Verification items for the finished model (mm, model axes). Face numbers are marked on the shaded views. A direction names the side the tool comes from. Round coordinates to 2 decimals unless told otherwise and drop trailing zeros. Write each loop counter-clockwise with the first axis right and the second up, starting at its lowest first coordinate (ties: lowest second). Pieces come first, ordered by that corner, then holes.
from build123d import *

# Parameters (mm, degrees)
F0_W     = 30
F0_H     = 12
F1_DEPTH = 5
F2_W     = 30
F2_H     = 7.47772
F3_DEPTH = 4
F4_W     = 15
F4_H     = 7.47772
F4_W_2   = 7
F5_DEPTH = 1.5
F6_W     = 13
F6_H     = 5.47772
F6_W_2   = 5
F7_DEPTH = 2.5
F8_R     = 1.5
F9_DEPTH = 2.5


with BuildPart() as f1:
    # F0 (on Front) → F1 (new body)
    with BuildSketch(Plane.XZ):
        Rectangle(F0_W, F0_H)
    extrude(amount=F1_DEPTH)

    # F2 (on face) → F3 (join)
    with BuildSketch(Plane.XZ.offset(5)):
        Rectangle(F2_W, F2_H)
    extrude(amount=F3_DEPTH)

    # F4 (on face) → F5 (join)
    with BuildSketch(Plane.XZ.offset(9)):
        with Locations((-7.5, 0)):
            Rectangle(F4_W, F4_H)
        with Locations((10.5, 0)):
            Rectangle(F4_W_2, F4_H)
    extrude(amount=F5_DEPTH)

    # F6 (on face) → F7 (cut)
    with BuildSketch(Plane.XZ.offset(10.5)):
        with Locations((-7.5, 0)):
            Rectangle(F6_W, F6_H)
        with Locations((10.5, 0)):
            Rectangle(F6_W_2, F6_H)
    extrude(amount=-F7_DEPTH, mode=Mode.SUBTRACT)

    # F8 (on face) → F9 (join)
    with BuildSketch(Plane(origin=(0, 0, 0), x_dir=(-1, 0, 0), z_dir=(0, 1, 0))):
        with BuildLine():
            Line((-15, 3.5), (-18.5, 3.5))
            ThreePointArc((-18.5, 3.5), (-22, 0), (-18.5, -3.5))
            Line((-18.5, -3.5), (-15, -3.5))
            Line((-15, -3.5), (-15, 3.5))
        make_face()
        with Locations((-18.5, 0)):
            Circle(F8_R, mode=Mode.SUBTRACT)
        with BuildLine():
            Line((18.5, 3.5), (15, 3.5))
            Line((15, 3.5), (15, -3.5))
            Line((15, -3.5), (18.5, -3.5))
            ThreePointArc((18.5, -3.5), (22, 0), (18.5, 3.5))
        make_face()
        with Locations((18.5, 0)):
            Circle(F8_R, mode=Mode.SUBTRACT)
    extrude(amount=-F9_DEPTH)


solid = f1.part
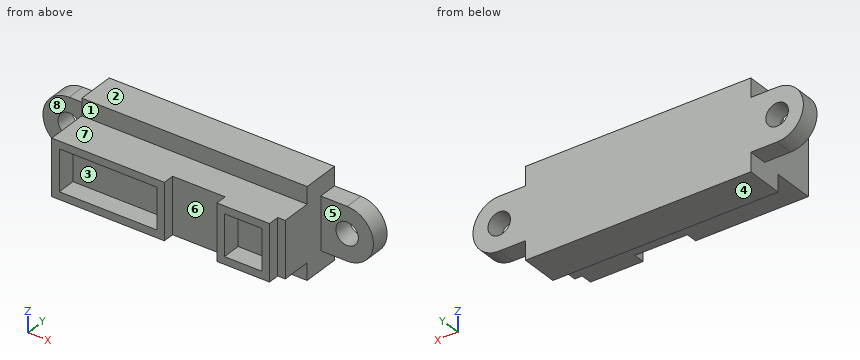
Q1. Material ranges on line 1 along X through (y, z) = (-1.75, -0.5); line 2 along Z through (x, y) = (18.5, -1.9); line 3 along X through (y, z) = (-5, -2), recorded low to high.
Recorded:
line 1: x = -21.96 to -19.91, -17.09 to 17.09, 19.91 to 21.96
line 2: z = -3.5 to -1.5, 1.5 to 3.5
line 3: x = -15 to 15
Q2. Release check for a two-part mould opening along Z. For the marked faces 1, 2, 3 and 4 record: released by +Z, released by -Z, zero draft, split by the parting line, or undercut.
Recorded:
face 1: zero draft
face 2: released by +Z
face 3: undercut
face 4: released by -Z
Q3. Sectioned sample at D-D (x = -6.5). Enter the section's corners in (y, z).
Recorded:
outline: (-10.5, -3.74) - (-5, -3.74) - (-5, -6) - (0, -6) - (0, 6) - (-5, 6) - (-5, 3.74) - (-10.5, 3.74) - (-10.5, 2.74) - (-8, 2.74) - (-8, -2.74) - (-10.5, -2.74) - close
Q4. Sectioned sample at A-A (z = 0). Give the number of separate pieces and of enclosed holes in the cut face, plus the area to 3 significant figures.
Recorded:
separate pieces: 3
enclosed holes: 0
area: 278 mm2
Q5. Depth check by flat-ended pin: P1, Ø3, axis at x = 11, z = 0, coming from the -Y side; P2, Ø1.2, axis at x = -5.5, y = -9.5, coming from the -Z side; P3, Ø1.6, axis at y = -10, z = 0.5, coming from the -X side; P4, Ø2.5, axis at x = 18.5, z = 0, coming from the +Y side. Enter the tip coordinate at first touch or a pass-through.
Recorded:
P1: stops at y = -8
P2: stops at z = -3.74
P3: stops at x = -15
P4: passes through
Q6. Sectioned sample at C-C (x = -19). Enter the section's corners in (y, z), plus the area to 3 significant figures.
Recorded:
outline: (-2.5, -3.46) - (0, -3.46) - (0, -1.41) - (-2.5, -1.41) - close; (-2.5, 1.41) - (0, 1.41) - (0, 3.46) - (-2.5, 3.46) - close
area: 10.2 mm2
Q7. Tool access check on the marked faces 5, 6, 7 and 8. Record the directions out of +Z, -Z, +X, -X, +Y, -Y that give a thin tool (end or side, any length) a straight path to the whole face; none if there is none.
Recorded:
face 5: +Z, -Z, +X, -Y
face 6: +Z, -Z, -Y
face 7: +Z, +X, -X, -Y
face 8: +Z, -Z, -X, -Y
Q8. Sectioned sample at B-B (y = -2). Enter the section's corners in (x, z).
Recorded:
outline: (-18.5, -3.5) - (-15, -3.5) - (-15, -6) - (15, -6) - (15, -3.5) - (18.5, -3.5) arc R3.5 ccw to (18.5, 3.5) - (15, 3.5) - (15, 6) - (-15, 6) - (-15, 3.5) - (-18.5, 3.5) arc R3.5 ccw to start; hole circle Ø3 at (-18.5, 0); hole circle Ø3 at (18.5, 0)
